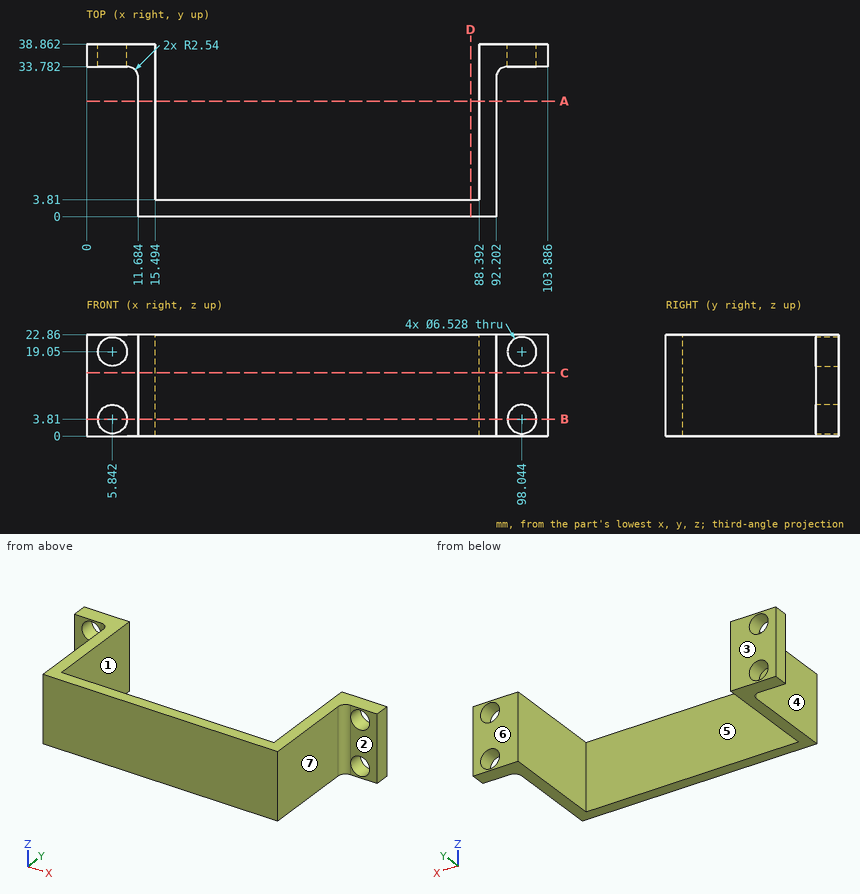
Could you check a few things on this drawing? It's one solid part, dimensions in mm from its lowest x, y, z. A direction names the side the tool comes from. Coordinates: 2 decimals unless noted, no trailing zeros. Loops run counter-clockwise (first coordinate to the right, second up) from the corner with the lowest first, then second, coordinate; pieces in that order, holes last. Notation, with made-up numbers: (-26, 61.5) - (8, 61.5) arc R26 ccw to (8, 85.5) - close; hole circle Ø10 at (0, 85). An arc over 180 degrees is marked (long way). Answer as a JSON object with one key per item and string values. Group by question number.
Item 1: If we section it at D-D (x = 86.5): List the corners of the cut face in (y, z) for me, plus the area to 3 significant figures.
Item 2: If we section it at C-C (z = 14.25): List the corners of the cut face in (x, y) for me.
Item 3: If we section it at B-B (z = 3.81): State how many separate pieces and enclosed holes the cut face has, plus the area to 3 significant figures.
Item 4: For pin 1 (6 mm diameter, centred on x = 37.5, z = 9, fed in from +Y); pin 2 (7.5 mm diameter, centred on x = 4, z = 8.5, fed in from -Y); pin 3 (1.5 mm diameter, centred on y = 31, z = 10.5, fed in from +X); pin 4 (4 mm diameter, centred on x = 98.044, z = 19.05, fed in from +Y), each with a flat end and sliding along its axis, tell me the tip position at first contact or that it passes through.
Item 5: If we mould it in two halves opening along X, with no side actions, what happens to the marked faces 5, 6 and 7? For each: released by +X, released by -X, zero draft, split by the parting line, or undercut.
Item 6: If we section it at A-A (y = 26): List the corners of the cut face in (x, z) for me, plus the area to 3 significant figures.
Item 7: On a 3-axis mill with a long thin cutter (end or side, diameter ignored), from which of +Z, -Z, +X, -X, +Y, -Y can I reach the whole of each face in a straight line? I mean the marked faces 1, 2, 3 and 4. Say none if no direction works.
Item 8: If I drill on L1, parallel to X at y = 35.45, z = 3.81; L2, parallel to X at y = 24.5, z = 18.5; L3, parallel to Y at x = 34, z = 6, over which ranges is the centre line in solid material (lowest first)? Write a range as from..to.
Returned:
{
 "1": {"outline": "(0, 0) - (3.81, 0) - (3.81, 22.86) - (0, 22.86) - close", "area": "87.1 mm²"},
 "2": {"outline": "(0, 33.78) - (9.14, 33.78) arc R2.54 cw to (11.68, 31.24) - (11.68, 0) - (92.2, 0) - (92.2, 31.24) arc R2.54 cw to (94.74, 33.78) - (103.89, 33.78) - (103.89, 38.86) - (88.39, 38.86) - (88.39, 3.81) - (15.49, 3.81) - (15.49, 38.86) - (0, 38.86) - close"},
 "3": {"separate pieces": "3", "enclosed holes": "0", "area": "629 mm²"},
 "4": {"pin 1": "stops at y = 3.81", "pin 2": "stops at y = 33.78", "pin 3": "stops at x = 92.25", "pin 4": "passes through"},
 "5": {"face 5": "undercut", "face 6": "zero draft", "face 7": "released by +X"},
 "6": {"outline": "(11.68, 0) - (15.49, 0) - (15.49, 22.86) - (11.68, 22.86) - close; (88.39, 0) - (92.2, 0) - (92.2, 22.86) - (88.39, 22.86) - close", "area": "174 mm²"},
 "7": {"face 1": "+Z, -Z, +Y", "face 2": "+Z, -Z, +X, -Y", "face 3": "+Z, -Z, +X, -X, +Y", "face 4": "+Z, -Z, -X, -Y"},
 "8": {"L1": "x = 0..2.58, 9.11..15.49, 88.39..94.78, 101.31..103.89", "L2": "x = 11.68..15.49, 88.39..92.2", "L3": "y = 0..3.81"}
}
